Check sheet for the drawn part. Datum: minimum x, y, z corner. Units: mm. A direction names the side the tool comes from. Round coordinates to 2 decimals unless told otherwise and drop trailing zeros. Write each loop counter-clockwise with the first axis right and the second up, starting at its lowest first coordinate (ties: lowest second). Pieces come first, ordered by that corner, then holes. Notation, with made-up numbers: (38.5, 29) - (52.5, 29) arc R17 cw to (52.5, 35) - close; hole circle Ø4 at (39, 35.25). An arc over 180 degrees is marked (long way). Answer as a JSON object with one key per item and string values. Group by question number.
Item 1: Gauge pin test, flat ends, axial feed: P1, Ø9, axis at x = 22, y = 15, coming from the -Z side; P2, Ø8, axis at x = 36.5, z = 29.5, coming from the +Y side; P3, Ø18.5, axis at y = 32.5, z = 35, coming from the +X side; P4, Ø4, axis at x = 51, y = 7, coming from the +Z side. Record the tip position at first contact, or that the pin passes through.
Item 2: Set-up check for the marked faces 1 and 2: record each of +Z, -Z, +X, -X, +Y, -Y from which the full face is reachable in a straight line by a thin tool's end or side.
Item 3: Sectioned sample at A-A on z = 12.5. Record the boundary of the cut face in (x, y).
Item 4: Thickness scan on line 1 (Y direction, x = 40, z = 13.5); line 2 (Z direction, x = 20, y = 16.5). Record the ranges inside material, lowest first.
Item 5: Sectioned sample at C-C on y = 8. Record the boundary of the cut face in (x, z).
Item 6: Sectioned sample at D-D on z = 55.5. Record the boundary of the cut face in (x, y).
Item 7: Sectioned sample at B-B on x = 49.5. Record the boundary of the cut face in (y, z).
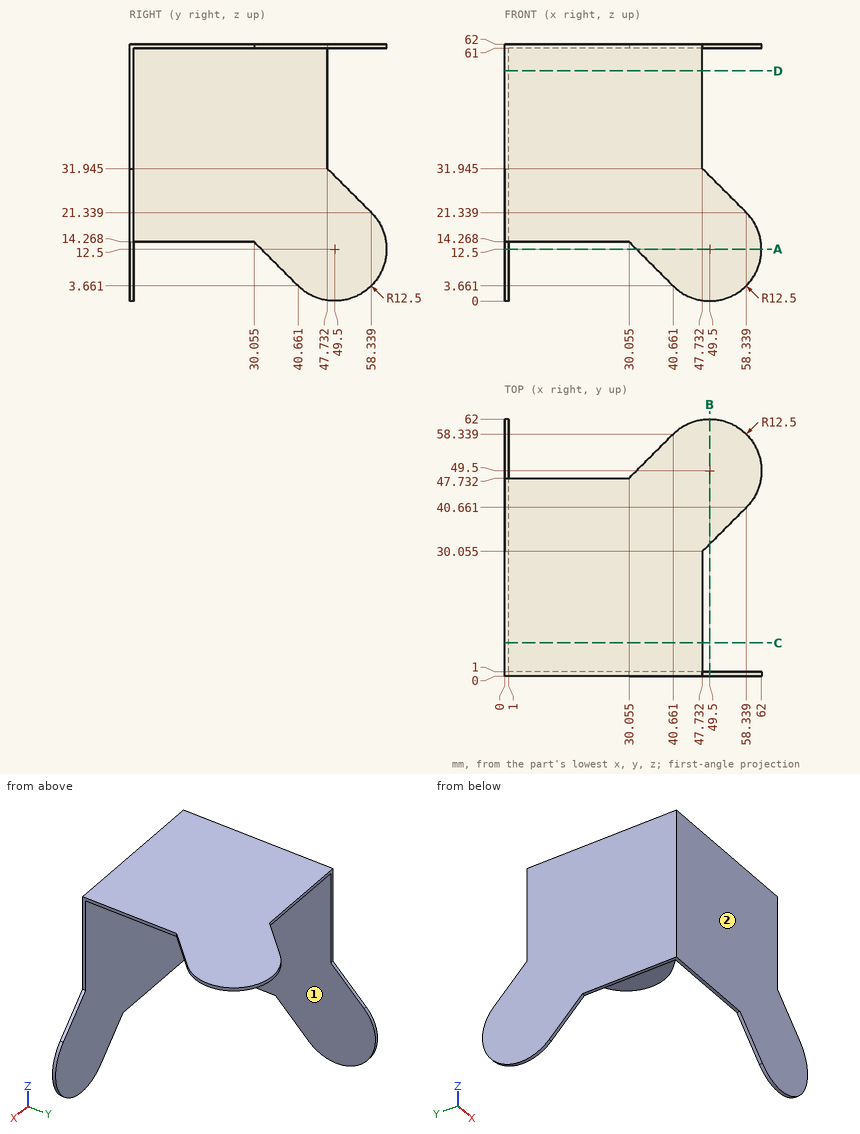
Completed:
{
 "1": {"P1": "z = 61", "P2": "y = 1", "P3": "x = 1", "P4": "through"},
 "2": {"face 1": "-Z, +X, +Y", "face 2": "+Z, -Z, +X, -X, -Y"},
 "3": {"outline": "(0, 31.82) - (1, 31.82) - (1, 62) - (0, 62) - close; (31.82, 0) - (62, 0) - (62, 1) - (31.82, 1) - close"},
 "4": {"line 1": "0 to 1", "line 2": "61 to 62"},
 "5": {"outline": "(0, 14.27) - (1, 14.27) - (1, 61) - (47.73, 61) - (47.73, 62) - (0, 62) - close"},
 "6": {"outline": "(0, 0) - (47.73, 0) - (47.73, 1) - (1, 1) - (1, 47.73) - (0, 47.73) - close"},
 "7": {"outline": "(0, 0) - (1, 0) - (1, 30.18) - (0, 30.18) - close; (31.82, 61) - (62, 61) - (62, 62) - (31.82, 62) - close"}
}
